Autodesk Inventor part; units mm, degrees
ref_plane "YZ Plane" through (0, 0, 0) normal (1, 0, 0) x (0, 1, 0)
ref_plane "XZ Plane" through (0, 0, 0) normal (0, 1, 0) x (-1, 0, 0)
ref_plane "XY Plane" through (0, 0, 0) normal (0, 0, 1) x (1, 0, 0)
sketch "スケッチ1" plane through (0, 0, 0) normal (0, 0, 1) x (1, 0, 0)
  circle A0 centre (-239, 204) radius 2.1 construction
  circle A1 centre (-239, -204) radius 2.1 construction
  circle A2 centre (239, -204) radius 2.1 construction
  circle A3 centre (239, 204) radius 2.1 construction
  circle A4 centre (-61, 204) radius 2.1 construction
  circle A5 centre (61, 204) radius 2.1 construction
  circle A6 centre (-50, -185) radius 2.1 construction
  circle A7 centre (-161.1336, -215) radius 2.1 construction
  circle A8 centre (50, -185) radius 2.1 construction
  circle A9 centre (150, -185) radius 2.1 construction
  circle A10 centre (161.1336, -215) radius 2.1 construction
  circle A11 centre (250, -185) radius 1.6 construction
  circle A12 centre (250, -215) radius 1.6 construction
  line L0 (239, 184) -> (239, -154) construction
  arc A13 (239, 184) -> (219, 204) centre (219, 184) ccw construction
  arc A14 (219, -174) -> (239, -154) centre (219, -154) ccw construction
  line L1 (219, -174) -> (-219, -174) construction
  line L2 (81, 204) -> (219, 204) construction
  line L3 (-239, -154) -> (-239, 184) construction
  arc A15 (-239, -154) -> (-219, -174) centre (-219, -154) ccw construction
  arc A16 (-219, 204) -> (-239, 184) centre (-219, 184) ccw construction
  line L4 (-219, 204) -> (-81, 204) construction
  arc A17 (-66.8579, 198.1421) -> (-55.1421, 198.1421) centre (-61, 204) ccw construction
  arc A18 (-66.8579, 198.1421) -> (-81, 204) centre (-81, 184) ccw construction
  arc A19 (-41, 204) -> (-55.1421, 198.1421) centre (-41, 184) ccw construction
  line L5 (-41, 204) -> (41, 204) construction
  arc A20 (55.1421, 198.1421) -> (41, 204) centre (41, 184) ccw construction
  arc A21 (55.1421, 198.1421) -> (66.8579, 198.1421) centre (61, 204) ccw construction
  arc A22 (81, 204) -> (66.8579, 198.1421) centre (81, 184) ccw construction
  circle A23 centre (-250, -215) radius 2.1 construction
  circle A24 centre (-239, 204) radius 10 construction
  circle A25 centre (-250, 215) radius 1.6 construction
  circle A26 centre (-250, 215) radius 5 construction
  circle A27 centre (-239, -204) radius 10 construction
  circle A28 centre (239, -204) radius 10 construction
  circle A29 centre (239, 204) radius 10 construction
  line L6 (245, -154) -> (245, 184) construction
  arc A30 (245, 184) -> (219, 210) centre (219, 184) ccw construction
  line L7 (219, 210) -> (81, 210) construction
  arc A31 (81, 210) -> (62.6152, 202.3848) centre (81, 184) ccw construction
  arc A32 (59.3848, 202.3848) -> (62.6152, 202.3848) centre (61, 204) ccw construction
  arc A33 (59.3848, 202.3848) -> (41, 210) centre (41, 184) ccw construction
  line L8 (41, 210) -> (-41, 210) construction
  arc A34 (-41, 210) -> (-59.3848, 202.3848) centre (-41, 184) ccw construction
  arc A35 (-62.6152, 202.3848) -> (-59.3848, 202.3848) centre (-61, 204) ccw construction
  arc A36 (-62.6152, 202.3848) -> (-81, 210) centre (-81, 184) ccw construction
  line L9 (-81, 210) -> (-219, 210) construction
  arc A37 (-219, 210) -> (-245, 184) centre (-219, 184) ccw construction
  line L10 (-245, 184) -> (-245, -154) construction
  arc A38 (-245, -154) -> (-219, -180) centre (-219, -154) ccw construction
  line L11 (-219, -180) -> (219, -180) construction
  arc A39 (219, -180) -> (245, -154) centre (219, -154) ccw construction
  circle A40 centre (250, -185) radius 5 construction
  circle A41 centre (250, 145) radius 2.1 construction
  circle A42 centre (250, 145) radius 5 construction
  circle A43 centre (150, -185) radius 5 construction
  circle A44 centre (61, 204) radius 5 construction
  line L12 (150.951, -180) -> (235.3288, -213.3018)
  line L13 (245, -154) -> (245, -185.5709)
  line L14 (245, -185.5709) -> (248.7426, -201.7457)
  arc A45 (235.3288, -213.3018) -> (248.7426, -201.7457) centre (239, -204) ccw
  line L15 (0, -174) -> (0, 204) construction
  line L16 (245, 145.1708) -> (248.9767, 203.3177)
  line L17 (238.7472, 213.9968) -> (80.3428, 209.9917)
  arc A46 (80.3428, 209.9917) -> (65.2441, 201.3566) centre (80.8062, 191.6636) ccw
  arc A47 (56.7774, 201.3225) -> (41, 210) centre (41, 191.3182) ccw
  arc A48 (56.7774, 201.3225) -> (65.2441, 201.3566) centre (61, 204) ccw
  line L18 (245, -154) -> (245, 145.1708)
  arc A49 (248.9767, 203.3177) -> (238.7472, 213.9968) centre (239, 204) ccw
  line L19 (-150.951, -180) -> (-235.3288, -213.3018)
  line L20 (-245, -154) -> (-245, -185.5709)
  line L21 (-245, -185.5709) -> (-248.7426, -201.7457)
  arc A50 (-248.7426, -201.7457) -> (-235.3288, -213.3018) centre (-239, -204) ccw
  line L22 (-245, 145.1708) -> (-248.9767, 203.3177)
  line L23 (-238.7472, 213.9968) -> (-80.3428, 209.9917)
  arc A51 (-65.2441, 201.3566) -> (-80.3428, 209.9917) centre (-80.8062, 191.6636) ccw
  arc A52 (-41, 210) -> (-56.7774, 201.3225) centre (-41, 191.3182) ccw
  arc A53 (-65.2441, 201.3566) -> (-56.7774, 201.3225) centre (-61, 204) ccw
  line L24 (-245, -154) -> (-245, 145.1708)
  arc A54 (-238.7472, 213.9968) -> (-248.9767, 203.3177) centre (-239, 204) ccw
  line L25 (-150.951, -180) -> (150.951, -180)
  line L26 (-41, 210) -> (41, 210)
  circle A55 centre (-239, -204) radius 2.1
  circle A56 centre (-239, 204) radius 2.1
  circle A57 centre (239, 204) radius 2.1
  circle A58 centre (239, -204) radius 2.1
  point P0 (0, 0)
  dimension "d0" = 20
  dimension "d1" = 10
  dimension "d2" = 6
  dimension "d3" = 10
  dimension "d4" = 4.2
extrude "押し出し1" add sketch "スケッチ1" along normal blind 3
sketch "スケッチ2" plane through (0, 0, 3) normal (0, 0, 1) x (1, 0, 0)
  circle A0 centre (-250, -200) radius 2.1 construction
  circle A1 centre (-250, -200) radius 5
  line L0 (41, 210) -> (-41, 210) construction
  line L1 (-150.951, -180) -> (150.951, -180) construction
  line L2 (0, 210) -> (0, -180) construction
  circle A2 centre (250, -200) radius 5
  point P0 (0, 0)
  dimension "d7" = 10
extrude "押し出し2" cut sketch "スケッチ2" against normal through all
fillet "フィレット1" radius 5 10 edges at (248.9603, -204.8907, 1.5) (247.3566, -195.7559, 1.5) (245, -185.5709, 1.5) (150.951, -180, 1.5) (245, 145.1708, 1.5) (-245, 145.1708, 1.5) (-245, -185.5709, 1.5) (-247.3566, -195.7559, 1.5) (-248.9603, -204.8907, 1.5) (-150.951, -180, 1.5)
properties part number "left_plate_02" material "ポリカーボネート、クリア"
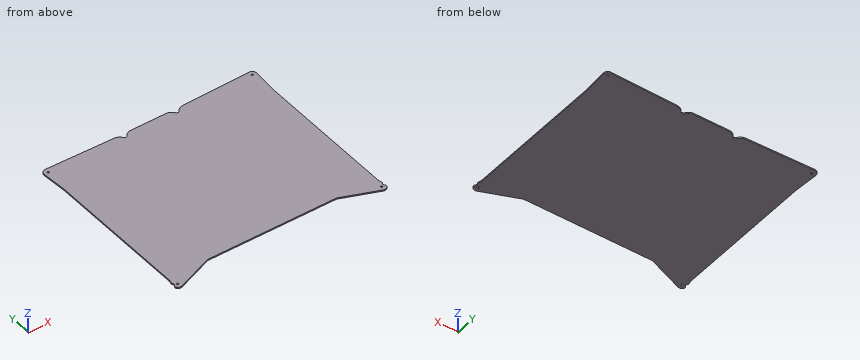
Here's how the part is built. I have some questions about the finished solid (model axes, mm). Give positions to 0.01 mm unless a question says otherwise; leave off trailing zeros. Order: outer loops, then holes, each group sorted by start corner. A loop starts at its lowest first (then second) coordinate and runs counter-clockwise, first axis right, second up. Notation, with made-up numbers: M 75,14 L 123,14 A21 cw 123,29 Z; hole C 15,27.25 d3. An arc over 180 degrees is marked long. Answer as a JSON object with one key per item and string values. Group by question number.
1) Suppose I cut it at C-C, the plane y = 129.5. Write out the boundary of the cut face in (x, z), plus the area to 3 significant figures.
2) Suppose I cut it at B-B, the plane x = -4.5. Write out the boundary of the cut face in (y, z), plus the area to 3 significant figures.
3) Please list where these lines run through material, in increasing order: L1, parallel to Y at x = 239, z = 0.6; L2, parallel to X at y = 204, z = 1.75; L3, parallel to Y at x = -28, z = 2.55. Write a range as [from, to].
4) I'm going to push flat-ended pins straight in: pin 1 Ø0.9 at (x, z) = (-22.5, 1) entering from -Y; pin 2 Ø1.5 at (y, z) = (-18.5, 1) entering from +X. Where does each tip first touch, or does it pass through?
5) Suppose I cut it at A-A, the plane z = 1. Count the separate pieces of the cut face and the enclosed holes in it, plus the area to 3 significant figures.
Results found:
{
 "1": {"outline": "M -245,0 L 245,0 L 245,3 L -245,3 Z", "area": "1,470 mm²"},
 "2": {"outline": "M -180,0 L 210,0 L 210,3 L -180,3 Z", "area": "1,170 mm²"},
 "3": {"L1": "[-214, -206.1], [-201.9, 201.9], [206.1, 214]", "L2": "[-249, -241.1], [-236.9, -67.24], [-54.72, 54.72], [67.24, 236.9], [241.1, 249]", "L3": "[-180, 210]"},
 "4": {"pin 1": "y = -180", "pin 2": "x = 245"},
 "5": {"separate pieces": "1", "enclosed holes": "4", "area": "195,000 mm²"}
}
